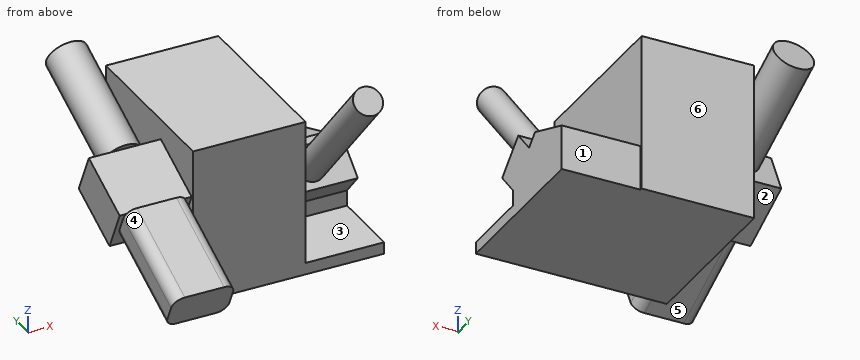
from build123d import *

# Parameters (mm, degrees)
F0_W      = 100
F0_H      = 150
F1_DEPTH  = 140
F2_W      = 70
F2_H      = 148
F3_DEPTH  = 85
F5_DEPTH  = 70
F6_R      = 12.5
F7_DEPTH  = 150
F9_DEPTH  = 64
F10_R     = 18
F11_DEPTH = 105
F13_DEPTH = 91


with BuildPart() as f1:
    # F0 (on Top) → F1 (new body)
    with BuildSketch(Plane.XY):
        Rectangle(F0_W, F0_H)
    extrude(amount=F1_DEPTH)

    # F2 (on Top) → F3 (join)
    with BuildSketch(Plane.XY):
        with Locations((85, -1)):
            Rectangle(F2_W, F2_H)
    extrude(amount=F3_DEPTH)

    # F4 (on face) → F5 (cut, through all)
    with BuildSketch(Plane.YZ.offset(120)):
        Polygon((27, 58), (73, 40), (73, 85), (-75, 85), (-75, 10.5), (-11, 10.5), (-11, 24.5), (-29.5162637007, 45.5035230037), (-1.7616083029, 69.9714428939), (16.7546553978, 48.9679198901), align=None)
    extrude(amount=-F5_DEPTH, mode=Mode.SUBTRACT)

    # F6 (on face) → F7 (join)
    with BuildSketch(Plane(origin=(0, -35.4800240514, 40.2459974314), x_dir=(1, 0, 0), z_dir=(0, -0.6612951322, 0.7501258216))):
        with Locations((85, 26.4503467009)):
            Circle(F6_R)
    extrude(amount=F7_DEPTH)

    # F8 (on face) → F9 (join)
    with BuildSketch(Plane(origin=(-50, 0, 0), x_dir=(0, -1, 0), z_dir=(-1, 0, 0))):
        Polygon((2, 85), (55, 60), (72.4913657042, 97.081695293), (19.4913657042, 122.081695293), align=None)
    extrude(amount=F9_DEPTH)

    # F10 (on face) → F11 (join)
    with BuildSketch(Plane(origin=(0, 31.1610366919, 14.6986022132), x_dir=(-1, 0, 0), z_dir=(0, 0.9044315925, 0.4266186757))):
        with Locations((82, 105.7299227149)):
            Circle(F10_R)
    extrude(amount=F11_DEPTH)

    # F12 (on face) → F13 (join)
    with BuildSketch(Plane(origin=(0, -21.8389633081, -10.3013977868), x_dir=(1, 0, 0), z_dir=(0, -0.9044315925, -0.4266186757))):
        with BuildLine():
            ThreePointArc((-109.5, 98.2299227149), (-106.5710678119, 91.158854903), (-99.5, 88.2299227149))
            Line((-99.5, 88.2299227149), (-64.5, 88.2299227149))
            ThreePointArc((-64.5, 88.2299227149), (-57.4289321881, 91.158854903), (-54.5, 98.2299227149))
            Line((-54.5, 98.2299227149), (-54.5, 113.2299227149))
            ThreePointArc((-54.5, 113.2299227149), (-57.4289321881, 120.3009905268), (-64.5, 123.2299227149))
            Line((-64.5, 123.2299227149), (-99.5, 123.2299227149))
            ThreePointArc((-99.5, 123.2299227149), (-106.5710678119, 120.3009905268), (-109.5, 113.2299227149))
            Line((-109.5, 113.2299227149), (-109.5, 98.2299227149))
        make_face()
    extrude(amount=F13_DEPTH)


solid = f1.part
Read the model definition and answer for the solid it produces. Units are mm, in the model's axes. Face numbers are marked on the shaded views. A direction names the side the tool comes from. Coordinates: 2 decimals unless noted, no trailing zeros. Loops run counter-clockwise (first coordinate to the right, second up) from the corner with the lowest first, then second, coordinate; pieces in that order, holes last.
Q1. Which of the six approach directions +Z, -Z, +X, -X, +Y, -Y give full straight-line access (tool end or side, diameter ignored) to the marked faces 1, 2 and 3?
Q2. The part is cut by section A-A on x = 101. Write down the section's boundary in (y, z), and give its area (3 significant figures).
Q3. The part is cut by section B-B on x = 26. Write down the section's boundary in (y, z).
Q4. The mould has two halves that part along Y. Classify the marked faces 4, 5 and 6: +Y half, -Y half, draft (parallel to the pull), parting line (faces both ways), or undercut.
Q5. Consider probe 1 along X at (y, z) = (23, 102); probe 2 along X at (y, z) = (-63.5, 79.5); probe 3 along Z at (x, y) = (8, -7.5). Determine where each line is inside the solid, lowest interval first.
Q6. The part is cut by section C-C on z = 130. Give the number of separate pieces and of enclosed holes in the cut face, and give its area (3 significant figures).
Q7. Each of these flat-tipped pins is pushed along its axis until it touches: pin 1 Ø19 at (x, y) = (81, -56.5) entering from +Z; pin 2 Ø8 at (x, z) = (25, 47.5) entering from +Y; pin 3 Ø12 at (x, y) = (-52.5, -29) entering from +Z; pin 4 Ø2 at (x, y) = (40, -72) entering from -Z. Where does it stop, or does it pass through?
Results below:
1. face 1: +Z, -Z, +X, +Y
1. face 2: -Z, -X, +Y
1. face 3: +X, -Y
2. outline: (-75, 0) - (73, 0) - (73, 40) - (27, 58) - (16.75, 48.97) - (-1.76, 69.97) - (-29.52, 45.5) - (-11, 24.5) - (-11, 10.5) - (-75, 10.5) - close
2. area: 5,530 mm2
3. outline: (-75, 0) - (75, 0) - (75, 140) - (-75, 140) - close
4. face 4: -Y half
4. face 5: undercut
4. face 6: +Y half
5. probe 1: x = -50 to 50
5. probe 2: x = -114 to 50
5. probe 3: z = 0 to 140
6. separate pieces: 3
6. enclosed holes: 0
6. area: 18,000 mm2
7. pin 1: stops at z = 133.28
7. pin 2: stops at y = 75
7. pin 3: stops at z = 140
7. pin 4: stops at z = 0
